from build123d import *

# Parameters (mm, degrees)
SKETCH1_R           = 1.25
BOSS_EXTRUDE1_DEPTH = 0.8
FILLET1_R           = 3


with BuildPart() as part:
    # Sketch1 → Boss-Extrude1 (new body, symmetric)
    with BuildSketch(Plane(origin=(0, 0, 0), x_dir=(1, 0, 0), z_dir=(0, 1, 0))):
        with BuildLine():
            Line((-67.314560089, 5), (-24.494897428, 5))
            ThreePointArc((-24.494897428, 5), (-12.5, -21.650635095), (16.577575733, -18.713203436))
            Line((16.577575733, -18.713203436), (37.987407064, -55.796119082))
            ThreePointArc((37.987407064, -55.796119082), (-33.75, -58.456714755), (-67.314560089, 5))
        make_face()
        with Locations((-62.5, 0)):
            Circle(SKETCH1_R, mode=Mode.SUBTRACT)
        with Locations((31.25, -54.126587737)):
            Circle(SKETCH1_R, mode=Mode.SUBTRACT)
        with Locations((2.216118041, -63.461317516)):
            Circle(SKETCH1_R, mode=Mode.SUBTRACT)
        with Locations((-30.785410886, -55.538351403)):
            Circle(SKETCH1_R, mode=Mode.SUBTRACT)
        with Locations((-39.961844832, -49.348768553)):
            Circle(SKETCH1_R, mode=Mode.SUBTRACT)
        with Locations((-50.377937108, -38.656350742)):
            Circle(SKETCH1_R, mode=Mode.SUBTRACT)
    extrude(amount=BOSS_EXTRUDE1_DEPTH, both=True)

    # Fillet1
    fillet1_edges = [part.edges().sort_by_distance(p)[0] for p in [
        (-67.314560089, 0, -5),
        (-24.494897428, 0, -5),
        (16.577575733, 0, 18.713203436),
        (37.987407064, 0, 55.796119082),
    ]]
    fillet(fillet1_edges, radius=FILLET1_R)


solid = part.part
Verification items for the finished model (mm, model axes). Coordinates: 2 decimals unless noted, no trailing zeros. Write each loop counter-clockwise with the first axis right and the second up, starting at its lowest first coordinate (ties: lowest second). Pieces come first, ordered by that corner, then holes. Notation, with made-up numbers: M -35.5,-14.75 L -27.5,-14.75 A31 cw -27.5,13.25 Z; hole C 29.5,20 d3. An arc over 180 degrees is marked long. Use a Markdown table: item, result.
Q1. Draft check along X on faces 1 (the face through (-32.86, 0.01, 58.96)), 2 (the face through (-12.84, 0.01, 21.45)), 3 (the face through (27.302, 0.011, 37.288)), 4 (the face through (31.827, -0.011, 55.236)). Enter one of: +X half, -X half, draft (parallel to the pull), parting line (faces both ways), or undercut.
Reply:
| item | result |
|---|---|
| face 1 | parting line |
| face 2 | undercut |
| face 3 | +X half |
| face 4 | undercut |
Q2. Sectioned sample at B-B, the plane x = 31.25. Record the boundary of the cut face in (y, z).
Reply:
| item | result |
|---|---|
| outline | M -0.8,44.13 L 0.8,44.13 L 0.8,52.88 L -0.8,52.88 Z; M -0.8,55.38 L 0.8,55.38 L 0.8,59.83 L -0.8,59.83 Z |
Q3. Sectioned sample at C-C, the plane y = -0.3. Record the boundary of the cut face in (x, z), plus the area to 3 significant figures.
Reply:
| item | result |
|---|---|
| outline | M -67.47,-2.09 A3 ccw -64.47,-5 L -27.93,-5 A3 ccw -24.94,-1.79 A25 cw 14.01,20.7 A3 ccw 18.29,21.69 L 36.56,53.33 A3 ccw 35.55,57.38 A67.5 ccw Z; hole C -62.5,0 d2.5; hole C -50.38,38.66 d2.5; hole C -39.96,49.35 d2.5; hole C -30.79,55.54 d2.5; hole C 2.22,63.46 d2.5; hole C 31.25,54.13 d2.5 |
| area | 4,500 mm² |
Q4. Sectioned sample at A-A, the plane z = 0. Record the boundary of the cut face in (x, y), plus the area to 3 significant figures.
Reply:
| item | result |
|---|---|
| outline | M -67.5,-0.8 L -63.75,-0.8 L -63.75,0.8 L -67.5,0.8 Z; M -61.25,-0.8 L -25,-0.8 L -25,0.8 L -61.25,0.8 Z |
| area | 64.0 mm² |
Q5. Thickness scan on line 1 (X direction, y = 0.05, z = 0); line 2 (X direction, y = 0.05, z = 55); line 3 (X direction, y = -0.15, z = 1). Record the ranges inside material, lowest first.
Reply:
| item | result |
|---|---|
| line 1 | x = -67.5 to -63.75, -61.25 to -25 |
| line 2 | x = -39.13 to -31.91, -29.66 to 30.36, 32.14 to 36.96 |
| line 3 | x = -67.49 to -63.25, -61.75 to -24.98 |
Q6. Sectioned sample at D-D, the plane x = -19.5. Record the boundary of the cut face in (y, z).
Reply:
| item | result |
|---|---|
| outline | M -0.8,15.64 L 0.8,15.64 L 0.8,64.62 L -0.8,64.62 Z |
